```python
from build123d import *

# Parameters (mm, degrees)
BOSS_EXTRUDE1_DEPTH = 3.5814
BOSS_EXTRUDE2_DEPTH = 3.5814
SKETCH4_R           = 8.1
CUT_EXTRUDE2_DEPTH  = 4.5814
CUT_EXTRUDE4_REACH  = 5.581
CUT_EXTRUDE5_REACH  = 5.581


with BuildPart() as part:
    # Sketch1 → Boss-Extrude1 (new body)
    with BuildSketch(Plane(origin=(0, 0, 0), x_dir=(1, 0, 0), z_dir=(0, 1, 0))):
        Polygon((-20.25, -13.1232), (20.25, -13.1232), (20.25, -2.125), (1.7907, -2.125), (1.7907, 2.125), (9.398, 2.125), (1.7907, 7.205), (-1.7907, 7.205), (-9.398, 2.125), (-1.7907, 2.125), (-1.7907, -2.125), (-20.25, -2.125), align=None)
    extrude(amount=BOSS_EXTRUDE1_DEPTH)

    # Sketch3 → Boss-Extrude2 (add)
    with BuildSketch(Plane(origin=(0, 3.5814, 0), x_dir=(1, 0, 0), z_dir=(0, 1, 0))):
        Polygon((-20.25, -2.125), (-20.25, -13.1232), (20.25, -13.1232), (20.25, -2.125), (1.7907, -2.125), (1.7907, 2.125), (9.398, 2.125), (1.7907, 7.205), (-1.7907, 7.205), (-9.398, 2.125), (-1.7907, 2.125), (-1.7907, -2.125), align=None)
        with BuildLine():
            Line((20.25, -13.1232), (-20.25, -13.1232))
            ThreePointArc((-20.25, -13.1232), (-13.331227209, -22.72714357), (-2.030596131, -19.205654357))
            ThreePointArc((-2.030596131, -19.205654357), (0, -18.191524388), (2.030596131, -19.205654357))
            ThreePointArc((2.030596131, -19.205654357), (13.331227209, -22.72714357), (20.25, -13.1232))
        make_face()
    extrude(amount=-BOSS_EXTRUDE2_DEPTH)

    # Sketch4 → Cut-Extrude2 (cut, through all)
    with BuildSketch(Plane(origin=(0, 3.5814, 0), x_dir=(1, 0, 0), z_dir=(0, 1, 0))):
        with Locations((-10.85, -13.1232)):
            Circle(SKETCH4_R)
        with Locations((10.85, -13.1232)):
            Circle(SKETCH4_R)
    extrude(amount=-CUT_EXTRUDE2_DEPTH, mode=Mode.SUBTRACT)

    # Sketch5 → Cut-Extrude4 (cut, up to next)
    with BuildSketch(Plane(origin=(0, 3.5814, 0), x_dir=(1, 0, 0), z_dir=(0, 1, 0)), mode=Mode.PRIVATE) as cut_extrude4_sk1:
        with BuildLine():
            Line((7, -5.996665078), (-7, -5.996665078))
            ThreePointArc((-7, -5.996665078), (-3.893168825, -8.974404994), (-2.75, -13.1232))
            Line((-2.75, -13.1232), (2.75, -13.1232))
            ThreePointArc((2.75, -13.1232), (3.893168825, -8.974404994), (7, -5.996665078))
        make_face()
    cut_extrude4_tool1 = extrude(cut_extrude4_sk1.sketch, amount=-CUT_EXTRUDE4_REACH, mode=Mode.PRIVATE) & part.part
    add(cut_extrude4_tool1.solids().sort_by_distance((0, 3.5814, 8.978273))[0], mode=Mode.SUBTRACT)

    # Sketch6 → Cut-Extrude5 (cut, up to next)
    with BuildSketch(Plane(origin=(0, 3.5814, 0), x_dir=(1, 0, 0), z_dir=(0, 1, 0)), mode=Mode.PRIVATE) as cut_extrude5_sk1:
        with BuildLine():
            Line((-9.2518, -2.125), (-20.25, -2.125))
            Line((-20.25, -2.125), (-20.25, -13.1232))
            ThreePointArc((-20.25, -13.1232), (-17.028701801, -5.346298199), (-9.2518, -2.125))
        make_face()
    cut_extrude5_tool1 = extrude(cut_extrude5_sk1.sketch, amount=-CUT_EXTRUDE5_REACH, mode=Mode.PRIVATE) & part.part
    add(cut_extrude5_tool1.solids().sort_by_distance((-17.793355, 3.5814, 4.581645))[0], mode=Mode.SUBTRACT)
    # Sketch6 → Cut-Extrude5 (cut, up to next)
    with BuildSketch(Plane(origin=(0, 3.5814, 0), x_dir=(1, 0, 0), z_dir=(0, 1, 0)), mode=Mode.PRIVATE) as cut_extrude5_sk2:
        with BuildLine():
            Line((20.25, -13.1232), (20.25, -2.125))
            Line((20.25, -2.125), (11.02035, -2.125))
            ThreePointArc((11.02035, -2.125), (17.636860555, -5.94429266), (20.25, -13.1232))
        make_face()
    cut_extrude5_tool2 = extrude(cut_extrude5_sk2.sketch, amount=-CUT_EXTRUDE5_REACH, mode=Mode.PRIVATE) & part.part
    add(cut_extrude5_tool2.solids().sort_by_distance((17.919058, 3.5814, 4.610875))[0], mode=Mode.SUBTRACT)


solid = part.part
```
Can you work these out from the model? Positions are in its coordinate system, mm. A direction names the side the tool comes from. Coordinates: 2 decimals unless noted, no trailing zeros. Order: outer loops, then holes, each group sorted by start corner. A loop starts at its lowest first (then second) coordinate and runs counter-clockwise, first axis right, second up. Notation, with made-up numbers: (11, 66) - (25, 66) arc R23 cw to (25, 101) - close; hole circle Ø2 at (85, -7.75). An arc over 180 degrees is marked (long way). Answer in a Markdown table with one row per item.
1. Suppose I cut it at C-C (x = -10.85). Please give me the cut outline in (y, z).
Reply:
| item | result |
|---|---|
| outline | (0, 2.24) - (3.58, 2.24) - (3.58, 5.02) - (0, 5.02) - close; (0, 21.22) - (3.58, 21.22) - (3.58, 23.22) - (0, 23.22) - close |
2. For pin 1 (1.5 mm diameter, centred on y = 2.5, z = 0, fed in from +X); pin 2 (4 mm diameter, centred on x = -3, z = 11, fed in from -Y); pin 3 (5 mm diameter, centred on x = 1, z = -1.5, fed in from -Y); pin 4 (1.5 mm diameter, centred on y = 0.5, z = 20, fed in from -X), each with a flat end and sliding along its axis, tell me the tip position at first contact or that it passes through.
Reply:
| item | result |
|---|---|
| pin 1 | stops at x = 1.79 |
| pin 2 | passes through |
| pin 3 | stops at y = 0 |
| pin 4 | stops at x = -18.19 |
3. Suppose I cut it at A-A (y = 1.45). Please give me the cut outline in (x, z) (3 decimals), and give its area (3 significant figures).
Reply:
| item | result |
|---|---|
| outline | (-20.25, 13.123) arc R10.998 ccw to (-9.252, 2.125) - (-1.791, 2.125) - (-1.791, -2.125) - (-9.398, -2.125) - (-1.791, -7.205) - (1.791, -7.205) - (9.398, -2.125) - (1.791, -2.125) - (1.791, 2.125) - (11.02, 2.125) arc R11.168 ccw to (20.25, 13.123) arc R10.125 ccw to (2.031, 19.206) arc R2.54 cw to (-2.031, 19.206) arc R10.125 ccw to start; hole (-7, 5.997) - (7, 5.997) arc R8.1 ccw (long way) to (2.75, 13.123) - (-2.75, 13.123) arc R8.1 ccw (long way) to start |
| area | 325 mm^2 |
4. If we mould it in two halves opening along Z, with no side actions, what happens to faces 1 (the cylindrical face through (-13.5, 1.82, 22.67)), 2 (the flat face through (-6, 2, -2.125)), 3 (the flat face through (-0.1, 0, 5.7))? For each: pulls with the +Z half, pulls with the -Z half, needs draft (parallel to the pull), parting line crosses it, or undercut.
Reply:
| item | result |
|---|---|
| face 1 | pulls with the +Z half |
| face 2 | undercut |
| face 3 | needs draft |
5. Suppose I cut it at D-D (x = -6.5). Please give me the cut outline in (y, z) (3 decimals), and give its area (3 significant figures).
Reply:
| item | result |
|---|---|
| outline | (0, -4.06) - (3.581, -4.06) - (3.581, -2.125) - (0, -2.125) - close; (0, 2.125) - (3.581, 2.125) - (3.581, 5.997) - (0, 5.997) - close; (0, 19.956) - (3.581, 19.956) - (3.581, 22.577) - (0, 22.577) - close |
| area | 30.2 mm^2 |
6. If I drill on line 1 along X through (y, z) = (2, 13.5); line 2 along X through (y, z) = (2.95, 16.5); line 3 along X through (y, z) = (3.3, 19.5), over which ranges is the centre line in solid material (lowest first)?
Reply:
| item | result |
|---|---|
| line 1 | x = -20.24 to -18.94, -2.76 to 2.76, 18.94 to 20.24 |
| line 2 | x = -19.67 to -18.21, -3.49 to 3.49, 18.21 to 19.67 |
| line 3 | x = -17.99 to -15.84, -5.86 to -2.26, 2.26 to 5.86, 15.84 to 17.99 |
7. For faces 4 (the flat face through (-1.791, 2, 0)), 5 (the flat face through (-0.1, 3.581, 5.7)), 6 (the flat face through (0, 2, -7.205)), 7 (the flat face through (1.791, 2, 0)), 8 (the flat face through (0, 2, 5.997)), which set-ups out of +Z, -Z, +X, -X, +Y, -Y let a thin tool reach every point of the face, with its end or its side?
Reply:
| item | result |
|---|---|
| face 4 | -X, +Y, -Y |
| face 5 | +Z, -Z, +X, -X, +Y |
| face 6 | -Z, +X, -X, +Y, -Y |
| face 7 | +X, +Y, -Y |
| face 8 | +Y, -Y |
8. Suppose I cut it at B-B (z = 11). Please give me the cut outline in (x, y), and give its area (3 significant figures).
Reply:
| item | result |
|---|---|
| outline | (-20.04, 0) - (-18.67, 0) - (-18.67, 3.58) - (-20.04, 3.58) - close; (18.67, 0) - (20.05, 0) - (20.05, 3.58) - (18.67, 3.58) - close |
| area | 9.87 mm^2 |
